Design review of the part built by this model. Coordinates are the model's own, in mm. Face numbers are marked on the shaded views. A direction names the side the tool comes from. Coordinates: 2 decimals unless noted, no trailing zeros. Order: outer loops, then holes, each group sorted by start corner. A loop starts at its lowest first (then second) coordinate and runs counter-clockwise, first axis right, second up. Notation, with made-up numbers: (39, -32) -> (78, -32) arc R33 cw to (78, -4) -> close; hole circle Ø8 at (85.25, 89.5). An arc over 180 degrees is marked (long way). Use a Markdown table: item, result. Add a question column.
Q1. Wall thickness on probe 1 along X at (y, z) = (33, -1); probe 2 along Y at (x, z) = (-2.5, -7.75); probe 3 along X at (y, z) = (52.5, -5.75): over which ranges is each line inside the solid? List them lowest first.
Q2. The part is to be moulded in two halves that separate along Y. For the marked faces 1, 2, 3 and 4, say which applies: pulls with the +Y half, pulls with the -Y half, needs draft (parallel to the pull), parting line crosses it, or undercut.
Q3. Add section C-C (y = 47.5). State the section outline as (x, z) points.
Q4. Machinability: for the marked faces 5, 6 and 7, which of the approach directions +Z, -Z, +X, -X, +Y, -Y give a long, thin tool a straight path to every point of the face, cutting with its end or side? Answer none if there is none.
Q5. Add section D-D (x = -8.5). State the section outline as (y, z) points.
Q6. Insertion check: pin 1 (2 mm diameter, centred on x = 14.5, z = -1.5, fed in from -Y); pin 2 (4 mm diameter, centred on x = 12, y = 38, fed in from -Z); pin 3 (0.8 mm diameter, centred on x = 16, z = -1.5, fed in from +Y); pin 4 (6 mm diameter, centred on x = -17, y = 17, fed in from -Z). Each pin has a flat end and moves straight along its axis. Give the tip position at first contact, or say it passes through.
Q7. Add section B-B (z = -4.75). State the section outline as (x, y) points, then the cut area to 3 significant figures.
Q8. Add section A-A (x = 0). State the section outline as (y, z) points, then the cut area to 3 significant figures.
from build123d import *

# Parameters (mm, degrees)
BOSS_EXTRUDE1_DEPTH  = 66.3956
BOSS_EXTRUDE2_DEPTH  = 1.27
SKETCH6_W            = 10
SKETCH6_H            = 15.618122384
SKETCH6_R            = 0.592132867
SKETCH6_W_2          = 1.524
BOSS_EXTRUDE4_DEPTH  = 2.54
M4_CLEARANCE_HOLE1_D = 4.8


with BuildPart() as part:
    # Sketch1 → Boss-Extrude1 (new body)
    with BuildSketch(Plane(origin=(0, 0, 0), x_dir=(1, 0, 0), z_dir=(0, 1, 0))):
        with BuildLine():
            Line((-11.557, 0), (-10.033, 0))
            ThreePointArc((-10.033, 0), (0, 10.033), (10.033, 0))
            Line((10.033, 0), (11.557, 0))
            ThreePointArc((11.557, 0), (0, 11.557), (-11.557, 0))
        make_face()
    extrude(amount=BOSS_EXTRUDE1_DEPTH)

    # Sketch2 → Boss-Extrude2 (add)
    with BuildSketch(Plane(origin=(0, 66.3956, 0), x_dir=(1, 0, 0), z_dir=(0, 1, 0))):
        with BuildLine():
            Line((-11.557, 0), (11.557, 0))
            ThreePointArc((11.557, 0), (0, 11.557), (-11.557, 0))
        make_face()
    boss_extrude2 = extrude(amount=BOSS_EXTRUDE2_DEPTH)

    # Mirror1: Boss-Extrude2 across plane
    add(boss_extrude2.mirror(Plane.ZX.offset(33.8328)))

    # Sketch6 → Boss-Extrude4 (add)
    # profile 1 of 4: a face of its own
    with BuildSketch(Plane.XY):
        with Locations((-16.557, 33.8328)):
            Rectangle(SKETCH6_W, SKETCH6_H)
        with Locations((-16.557, 33.8328)):
            Circle(SKETCH6_R, mode=Mode.SUBTRACT)
    # profile 2 of 4: a face of its own
    with BuildSketch(Plane.XY):
        with Locations((-10.795, 33.8328)):
            Rectangle(SKETCH6_W_2, SKETCH6_H)
    # profile 3 of 4: a face of its own
    with BuildSketch(Plane.XY):
        with Locations((10.795, 33.8328)):
            Rectangle(SKETCH6_W_2, SKETCH6_H)
    # profile 4 of 4: a face of its own
    with BuildSketch(Plane.XY):
        with Locations((16.557, 33.8328)):
            Rectangle(SKETCH6_W, SKETCH6_H)
        with Locations((16.557, 33.8328)):
            Circle(SKETCH6_R, mode=Mode.SUBTRACT)
    extrude(amount=-BOSS_EXTRUDE4_DEPTH)

    # M4 Clearance Hole1 (through all)
    with Locations(Plane(origin=(0, 0, -2.54), x_dir=(-1, 0, 0), z_dir=(0, 0, -1))):
        with Locations((-16.557, 33.8328), (16.557, 33.8328)):
            Hole(M4_CLEARANCE_HOLE1_D / 2)


solid = part.part
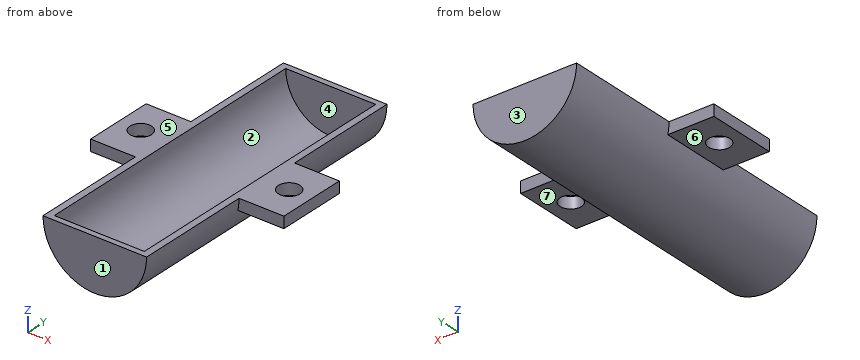
Established:
| question | item | result |
|---|---|---|
| 1 | probe 1 | -21.56 to -18.81, -14.31 to -9.98, 9.98 to 14.31, 18.81 to 21.56 |
| 1 | probe 2 | 0 to 1.27, 66.4 to 67.67 |
| 1 | probe 3 | -10.03 to -8.22, 8.22 to 10.03 |
| 2 | face 1 | pulls with the -Y half |
| 2 | face 2 | undercut |
| 2 | face 3 | pulls with the +Y half |
| 2 | face 4 | undercut |
| 3 | outline | (-11.56, 0) arc R11.56 ccw to (11.56, 0) -> (10.03, 0) arc R10.03 cw to (-10.03, 0) -> close |
| 4 | face 5 | +Z, +X, -X, +Y, -Y |
| 4 | face 6 | -Z, -X, +Y, -Y |
| 4 | face 7 | -Z, +X, +Y, -Y |
| 5 | outline | (0, -7.83) -> (67.67, -7.83) -> (67.67, 0) -> (66.4, 0) -> (66.4, -5.33) -> (1.27, -5.33) -> (1.27, 0) -> (0, 0) -> close |
| 6 | pin 1 | y = 26.02 |
| 6 | pin 2 | z = -5.79 |
| 6 | pin 3 | y = 41.64 |
| 6 | pin 4 | through |
| 7 | outline | (-10.54, 0) -> (10.54, 0) -> (10.54, 67.67) -> (-10.54, 67.67) -> close; hole (-8.84, 1.27) -> (8.84, 1.27) -> (8.84, 66.4) -> (-8.84, 66.4) -> close |
| 7 | area | 275 mm^2 |
| 8 | outline | (0, -11.56) -> (67.67, -11.56) -> (67.67, 0) -> (66.4, 0) -> (66.4, -10.03) -> (1.27, -10.03) -> (1.27, 0) -> (0, 0) -> close |
| 8 | area | 129 mm^2 |
